from build123d import *

# Parameters (mm, degrees)
CHAMFER_1_SIZE = 1


with BuildPart() as part:
    # 草图1 → 旋转1 (revolve)
    with BuildSketch(Plane.XY, mode=Mode.PRIVATE) as revolve_1_sk:
        with BuildLine():
            Line((-10.5, 41.5), (-1.717556404, 41.5))
            ThreePointArc((-1.717556404, 41.5), (0, 42), (1.717556404, 41.5))
            Line((1.717556404, 41.5), (10.5, 41.5))
            Line((10.5, 41.5), (10.5, 48.885069295))
            ThreePointArc((10.5, 48.885069295), (0, 50), (-10.5, 48.885069295))
            Line((-10.5, 48.885069295), (-10.5, 41.5))
        make_face()
    revolve(revolve_1_sk.sketch.rotate(Axis((-55.270843916, 0, 0), (1, 0, 0)), 90), axis=Axis((-55.270843916, 0, 0), (1, 0, 0)))

    # 倒角1
    chamfer_1_edges = [part.edges().sort_by_distance(p)[0] for p in [
        (10.5, 0, -41.5),
        (-10.5, 0, -41.5),
    ]]
    chamfer(chamfer_1_edges, length=CHAMFER_1_SIZE)


solid = part.part
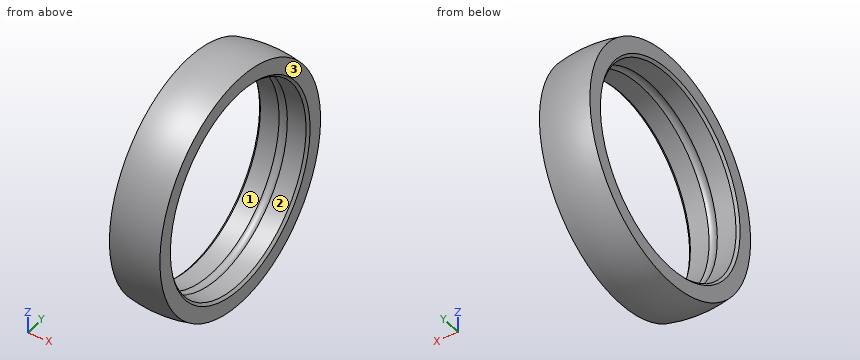
Design review of the part built by this model. Coordinates are the model's own, in mm. Face numbers are marked on the shaded views. Round coordinates to 2 decimals unless told otherwise and drop trailing zeros. Write each loop counter-clockwise with the first axis right and the second up, starting at its lowest first coordinate (ties: lowest second). Pieces come first, ordered by that corner, then holes. Notation, with made-up numbers: (17, 36.25) -> (34, 36.25) arc R20 cw to (34, 41.25) -> close; hole circle Ø3 at (-5, 87.5). An arc over 180 degrees is marked (long way). One line per item, written item: value. Start each with the question number.
Q1. Add section D-D (x = -6.25). Give the boundary of the cut face in (y, z), then the cut area to 3 significant figures.
Q2. Add section C-C (x = 3.5). Give the boundary of the cut face in (y, z).
Q3. The part is to be moulded in two halves that separate along Z. For the marked faces 1, 2 and 3, say which applies: pulls with the +Z half, pulls with the -Z half, needs draft (parallel to the pull), parting line crosses it, or undercut.
Q4. To check wall thickness, follow probe 1 along Y at (x, z) = (-1.75, 25); probe 2 along Y at (x, z) = (3.75, 29); probe 3 along Z at (x, y) = (5.75, 15.5). State the ranges of each line that lie inside material, in increasing order.
Q5. Add section A-A (z = 0). Give the boundary of the cut face in (x, y), then the cut area to 3 significant figures.
Q6. Insertion check: P1, Ø5, axis at x = -3, y = 25, coming from the +Z side; P2, Ø12, axis at x = 3.5, z = -18.5, coming from the -Y side; P3, Ø1, axis at x = -3.5, y = 29, coming from the -Z side. Each pin has a flat end and moves straight along its axis. Give the tip position at first contact, or say it passes through.
Response:
1. outline: circle Ø99.22 at (0, 0); hole circle Ø83 at (0, 0)
1. area: 2,320 mm^2
2. outline: circle Ø99.75 at (0, 0); hole circle Ø83 at (0, 0)
3. face 1: undercut
3. face 2: undercut
3. face 3: needs draft
4. probe 1: y = -43.27 to -33.12, 33.12 to 43.27
4. probe 2: y = -40.56 to -29.69, 29.69 to 40.56
4. probe 3: z = -47.19 to -38.5, 38.5 to 47.19
5. outline: (-10.5, -48.89) arc R50 ccw to (10.5, -48.89) -> (10.5, -42.5) -> (9.5, -41.5) -> (1.72, -41.5) arc R3.2 cw to (-1.72, -41.5) -> (-9.5, -41.5) -> (-10.5, -42.5) -> close; (-10.5, 42.5) -> (-9.5, 41.5) -> (-1.72, 41.5) arc R3.2 cw to (1.72, 41.5) -> (9.5, 41.5) -> (10.5, 42.5) -> (10.5, 48.89) arc R50 ccw to (-10.5, 48.89) -> close
5. area: 337 mm^2
6. P1: stops at z = 44.56
6. P2: stops at y = -48.33
6. P3: stops at z = -40.94
